from build123d import *

# Parameters (mm, degrees)
EXTRUDE_THIN1_DEPTH = 571.5
FILLET1_R           = 3.048


with BuildPart() as part:
    # Sketch1 → Extrude-Thin1 (new body)
    with BuildSketch(Plane.XY):
        with BuildLine():
            Line((0, 38.166088515), (-7.14375, 38.166088515))
            ThreePointArc((-7.14375, 38.166088515), (-9.525, 40.547338515), (-11.90625, 38.166088515))
            Line((-11.90625, 38.166088515), (-15.715448212, 38.166088515))
            Line((-15.715448212, 38.166088515), (-26.940768363, 26.940768363))
            Line((-26.940768363, 26.940768363), (-29.096029832, 29.096029832))
            Line((-29.096029832, 29.096029832), (-16.97797115, 41.214088515))
            Line((-16.97797115, 41.214088515), (-14.017933514, 41.214088515))
            ThreePointArc((-14.017933514, 41.214088515), (-9.525, 43.595338515), (-5.032066486, 41.214088515))
            Line((-5.032066486, 41.214088515), (0, 41.214088515))
            Line((0, 41.214088515), (0, 38.166088515))
        make_face()
    extrude(amount=-EXTRUDE_THIN1_DEPTH)

    # Fillet1
    fillet1_edges = [part.edges().sort_by_distance(p)[0] for p in [
        (-16.97797115, 41.214088515, -285.75),
        (-7.14375, 38.166088515, -285.75),
        (-11.90625, 38.166088515, -285.75),
    ]]
    fillet(fillet1_edges, radius=FILLET1_R)

    # Mirror1: part across plane


with BuildPart() as part_1:
    add(part.part)
    add(part.part.mirror(Plane(origin=(0, 41.214088515, -571.5), x_dir=(0, 0, 1), z_dir=(-1, 0, 0))))


solid = part_1.part
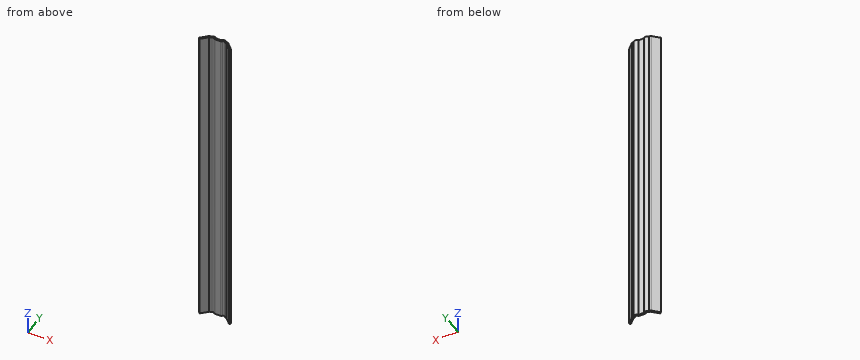
Can you work these out from the model? Positions are in its coordinate system, mm. Round coordinates to 2 decimals unless told otherwise and drop trailing zeros. Loops run counter-clockwise (first coordinate to the right, second up) from the corner with the lowest first, then second, coordinate; pieces in that order, holes last. Notation, with made-up numbers: (16.25, 87) - (44.25, 87) arc R32 ccw to (44.25, 113) - close; hole circle Ø1 at (-29, -25). An arc over 180 degrees is marked (long way). Write item = value, one per line. Start each with the question number.
(1) For P1, Ø5, axis at y = 32, z = -316, coming from the -X side; P2, Ø5, axis at y = 41.5, z = -433.5, coming from the -X side; P3, Ø6, axis at y = 36, z = -85.5, coming from the +X side, each with a flat end and sliding along its axis, tell me the tip position at first contact or that it passes through.
(2) If I drill on probe 1 along X at (y, z) = (41.25, -420); probe 2 along Y at (x, z) = (3, -181); probe 3 along X at (y, z) = (38.75, -27.5), over which ranges is the centre line in solid material (lowest first)? Write a range as [from, to].
(3) If we section it at B-B (y = 32.5): Please give me the cut outline in (x, z).
(4) If we section it at A-A (z = -185.5): Please give me the cut outline in (x, y) (1 decimal), and give its area (3 significant figures).
Ans:
q1.P1 = -28.69
q1.P2 = -19.19
q1.P3 = 25.19
q2.probe_1 = [-13.99, -5.06], [5.06, 13.99]
q2.probe_2 = [38.17, 41.21]
q2.probe_3 = [-19.44, -12.22], [-6.83, 6.83], [12.22, 19.44]
q3.outline = (-25.69, -571.5) - (-21.38, -571.5) - (-21.38, 0) - (-25.69, 0) - close; (21.38, -571.5) - (25.69, -571.5) - (25.69, 0) - (21.38, 0) - close
q4.outline = (-29.1, 29.1) - (-26.9, 26.9) - (-15.7, 38.2) - (-14, 38.2) arc R3 ccw to (-11.5, 39.5) arc R2.4 cw to (-7.6, 39.5) arc R3 ccw to (-5, 38.2) - (5, 38.2) arc R3 ccw to (7.6, 39.5) arc R2.4 cw to (11.5, 39.5) arc R3 ccw to (14, 38.2) - (15.7, 38.2) - (26.9, 26.9) - (29.1, 29.1) - (17.9, 40.3) arc R3 ccw to (15.7, 41.2) - (14, 41.2) arc R5.4 ccw to (5, 41.2) - (-5, 41.2) arc R5.4 ccw to (-14, 41.2) - (-15.7, 41.2) arc R3 ccw to (-17.9, 40.3) - close
q4.area = 210 mm²
